Geometry: final body of the model. Coordinates: model frame, mm. A direction names the side the tool comes from. Give positions to 0.01 mm unless a question says otherwise; leave off trailing zeros. Write each loop counter-clockwise with the first axis right and the second up, starting at its lowest first coordinate (ties: lowest second). Pieces come first, ordered by that corner, then holes. Notation, with made-up numbers: M 85,-36 L 144,-36 A9 cw 144,-27 Z; hole C 6,-29 d7. An arc over 180 degrees is marked long. Use a Markdown table: item, result. Add a question column.
1) Section C-C on z = 2.2. Return the cut outline in (x, y), then the cut area to 3 significant figures.
2) Pin query (flat end, axial travel): pin 1 (5 mm diameter, centred on x = -80.5, y = 20.5, fed in from -Z); pin 2 (1.5 mm diameter, centred on x = -10.5, z = 1.5, fed in from -Y). Return the tip coordinate at first contact, or that it passes through.
3) Set-up query: faces 3 (the flat face through (2, 1, 0)), 4 (the flat face through (-93.329, -87.884, 1.479)). Return all of +Z, -Z, +X, -X, +Y, -Y with unobstructed straight access to the full face (end or side cutting, diameter ignored); none if empty.
4) Section B-B on x = 14. Return the cut outline in (y, z), then the cut area to 3 significant figures.
5) Section A-A on y = -82. Return the cut outline in (x, z).
6) Section D-D on x = 73. Return the cut outline in (y, z), then the cut area to 3 significant figures.
7) Line query: line 1 (Y direction, x = 16.5, z = 1.1); line 2 (X direction, y = -21.5, z = 2.1); line 3 (X direction, y = -84, z = 1.3). Output: solid intervals per line, ascending.
8) Draft query along X for faces 1 (the flat face through (93.62, -88.19, 1.48)), 2 (the flat face through (2, 1, 3)). Return one class per face: +X half, -X half, draft (parallel to the pull), parting line (faces both ways), or undercut.
```python
from build123d import *

# Parameters (mm, degrees)
SKETCH1_W           = 140
SKETCH1_H           = 20
BOSS_EXTRUDE1_DEPTH = 3


with BuildPart() as part:
    # Sketch1 → Boss-Extrude1 (new body)
    with BuildSketch(Plane.XY):
        with BuildLine():
            Line((-124, -99), (-124, 99))
            Line((-124, 99), (124, 99))
            Line((124, 99), (124, -99))
            Line((124, -99), (104, -99))
            Line((104, -99), (82.951694449, -77.074681718))
            ThreePointArc((82.951694449, -77.074681718), (79.65871509, -74.800728757), (75.737821239, -74))
            Line((75.737821239, -74), (-75.737821239, -74))
            ThreePointArc((-75.737821239, -74), (-79.65871509, -74.800728757), (-82.951694449, -77.074681718))
            Line((-82.951694449, -77.074681718), (-104, -99))
            Line((-104, -99), (-124, -99))
        make_face()
        with Locations((0, -19)):
            Rectangle(SKETCH1_W, SKETCH1_H, mode=Mode.SUBTRACT)
    extrude(amount=BOSS_EXTRUDE1_DEPTH)


solid = part.part
```
Found:
| question | item | result |
|---|---|---|
| 1 | outline | M -124,-99 L -104,-99 L -82.95,-77.07 A10 cw -75.74,-74 L 75.74,-74 A10 cw 82.95,-77.07 L 104,-99 L 124,-99 L 124,99 L -124,99 Z; hole M -70,-29 L 70,-29 L 70,-9 L -70,-9 Z |
| 1 | area | 41,700 mm² |
| 2 | pin 1 | z = 0 |
| 2 | pin 2 | y = -74 |
| 3 | face 3 | -Z, +X, -X, +Y, -Y |
| 3 | face 4 | +Z, -Z, -Y |
| 4 | outline | M -74,0 L -29,0 L -29,3 L -74,3 Z; M -9,0 L 99,0 L 99,3 L -9,3 Z |
| 4 | area | 459 mm² |
| 5 | outline | M -124,0 L -87.68,0 L -87.68,3 L -124,3 Z; M 87.68,0 L 124,0 L 124,3 L 87.68,3 Z |
| 6 | outline | M -74,0 L 99,0 L 99,3 L -74,3 Z |
| 6 | area | 519 mm² |
| 7 | line 1 | -74 to -29, -9 to 99 |
| 7 | line 2 | -124 to -70, 70 to 124 |
| 7 | line 3 | -124 to -89.6, 89.6 to 124 |
| 8 | face 1 | undercut |
| 8 | face 2 | draft |
